```python
from build123d import *

# Parameters (mm, degrees)
SKETCH1_W                    = 44
SKETCH1_H                    = 90
BASE_FLANGE1_DEPTH           = 1.5
EDGE_FLANGE1_STRIP_W         = 7.4732
EDGE_FLANGE1_STRIP_H         = 1.5
EDGE_FLANGE1_STRIP_CUT_DEPTH = 90
EDGE_FLANGE1_DEPTH           = 90
EDGE_FLANGE2_STRIP_W         = 7.4732
EDGE_FLANGE2_STRIP_H         = 1.5
EDGE_FLANGE2_STRIP_CUT_DEPTH = 90
EDGE_FLANGE2_DEPTH           = 90
SKETCH12_R                   = 4.5
SKETCH12_R_2                 = 1.5
CUT_EXTRUDE4_DEPTH           = 68.906185285
SKETCH13_R                   = 4.5
SKETCH13_R_2                 = 1.5
CUT_EXTRUDE5_DEPTH           = 10
LPATTERN1_COUNT              = 2
LPATTERN1_PITCH              = 30
LPATTERN1_COL_COUNT          = 2
LPATTERN1_COL_PITCH          = 30
FILLET1_R                    = 2


# Sheet-metal steps are written as plain solids
with BuildPart() as part:
    # Sketch1 → Base-Flange1 (new body)
    with BuildSketch(Plane(origin=(0, 0, 0), x_dir=(1, 0, 0), z_dir=(0, 1, 0))):
        with Locations((-22, 0)):
            Rectangle(SKETCH1_W, SKETCH1_H)
    extrude(amount=BASE_FLANGE1_DEPTH)

    # Edge-Flange1 strip (across the edge) → Edge-Flange1 strip cut (cut)
    with BuildSketch(Plane(origin=(0, 1.5, 45), x_dir=(-1, 0, 0), z_dir=(0, 0, -1))):
        with Locations((-1.5, -0.75)):
            Rectangle(EDGE_FLANGE1_STRIP_W, EDGE_FLANGE1_STRIP_H)
    extrude(amount=EDGE_FLANGE1_STRIP_CUT_DEPTH, mode=Mode.SUBTRACT)

    # Edge-Flange1 section (across the edge) → Edge-Flange1 (add)
    with BuildSketch(Plane(origin=(0, 1.5, 45), x_dir=(-1, 0, 0), z_dir=(0, 0, -1))):
        with BuildLine():
            Line((0, 0.7366), (0, 24))
            Line((0, 24), (1.5, 24))
            Line((1.5, 24), (1.5, 0.7366))
            ThreePointArc((1.5, 0.7366), (1.715745145, 0.215745145), (2.2366, 0))
            Line((2.2366, 0), (2.2366, -1.5))
            ThreePointArc((2.2366, -1.5), (0.655084973, -0.844915027), (0, 0.7366))
        make_face()
    extrude(amount=EDGE_FLANGE1_DEPTH)

    # Edge-Flange2 strip (across the edge) → Edge-Flange2 strip cut (cut)
    with BuildSketch(Plane(origin=(-1.5, 25.5, 45), x_dir=(0, -1, 0), z_dir=(0, 0, -1))):
        with Locations((-1.5, -0.75)):
            Rectangle(EDGE_FLANGE2_STRIP_W, EDGE_FLANGE2_STRIP_H)
    extrude(amount=EDGE_FLANGE2_STRIP_CUT_DEPTH, mode=Mode.SUBTRACT)

    # Edge-Flange2 section (across the edge) → Edge-Flange2 (add)
    with BuildSketch(Plane(origin=(-1.5, 25.5, 45), x_dir=(0, -1, 0), z_dir=(0, 0, -1))):
        with BuildLine():
            Line((0, 0.7366), (0, 42.5))
            Line((0, 42.5), (1.5, 42.5))
            Line((1.5, 42.5), (1.5, 0.7366))
            ThreePointArc((1.5, 0.7366), (1.715745145, 0.215745145), (2.2366, 0))
            Line((2.2366, 0), (2.2366, -1.5))
            ThreePointArc((2.2366, -1.5), (0.655084973, -0.844915027), (0, 0.7366))
        make_face()
    extrude(amount=EDGE_FLANGE2_DEPTH)

    # Sketch12 → Cut-Extrude4 (cut, through all)
    with BuildSketch(Plane(origin=(0, 0, 0), x_dir=(1, 0, 0), z_dir=(0, 1, 0))):
        with Locations((-31, 35)):
            Circle(SKETCH12_R)
        with Locations((-31, 42)):
            Circle(SKETCH12_R_2)
        with Locations((-31, 28)):
            Circle(SKETCH12_R_2)
        with Locations((-24, 35)):
            Circle(SKETCH12_R_2)
        with Locations((-38, 35)):
            Circle(SKETCH12_R_2)
        with Locations((-31, 0)):
            Circle(SKETCH12_R)
        with Locations((-31, 7)):
            Circle(SKETCH12_R_2)
        with Locations((-31, -7)):
            Circle(SKETCH12_R_2)
        with Locations((-24, 0)):
            Circle(SKETCH12_R_2)
        with Locations((-38, 0)):
            Circle(SKETCH12_R_2)
        with Locations((-31, -35)):
            Circle(SKETCH12_R)
        with Locations((-31, -28)):
            Circle(SKETCH12_R_2)
        with Locations((-24, -35)):
            Circle(SKETCH12_R_2)
        with Locations((-38, -35)):
            Circle(SKETCH12_R_2)
        with Locations((-31, -42)):
            Circle(SKETCH12_R_2)
    extrude(amount=CUT_EXTRUDE4_DEPTH, mode=Mode.SUBTRACT)

    # Sketch13 → Cut-Extrude5 (cut)
    with BuildSketch(Plane.ZY.offset(1.5)):
        with Locations(Location((0, 12.75, 0), (0, 0, 270))):
            Circle(SKETCH13_R)
        with Locations(Location((0, 19.75, 0), (0, 0, 270))):
            Circle(SKETCH13_R_2)
        with Locations(Location((0, 5.75, 0), (0, 0, 270))):
            Circle(SKETCH13_R_2)
        with Locations(Location((7, 12.75, 0), (0, 0, 270))):
            Circle(SKETCH13_R_2)
        with Locations(Location((-7, 12.75, 0), (0, 0, 270))):
            Circle(SKETCH13_R_2)
    cut_extrude5 = extrude(amount=-CUT_EXTRUDE5_DEPTH, mode=Mode.SUBTRACT)

    # LPattern1: Cut-Extrude5 ×2
    with Locations(*[(0, 0, -i * LPATTERN1_PITCH) for i in range(1, LPATTERN1_COUNT)]):
        add(cut_extrude5, mode=Mode.SUBTRACT)

    # LPattern1 col: Cut-Extrude5 ×2
    with Locations(*[(0, 0, i * LPATTERN1_COL_PITCH) for i in range(1, LPATTERN1_COL_COUNT)]):
        add(cut_extrude5, mode=Mode.SUBTRACT)

    # Fillet1
    fillet1_edges = [part.edges().sort_by_distance(p)[0] for p in [
        (-44, 24.75, 45),
        (-44, 24.75, -45),
        (-44, 0.75, 45),
        (-44, 0.75, -45),
    ]]
    fillet(fillet1_edges, radius=FILLET1_R)


solid = part.part
```
Could you check a few things on this model? Use its own coordinates, in mm. Round coordinates to 2 decimals unless told otherwise and drop trailing zeros. Order: outer loops, then holes, each group sorted by start corner. A loop starts at its lowest first (then second) coordinate and runs counter-clockwise, first axis right, second up. Notation, with made-up numbers: (-4.75, 57) -> (23.25, 57) arc R12 ccw to (23.25, 67) -> close; hole circle Ø3 at (-26, -26.75). An arc over 180 degrees is marked (long way). One line per question, with ' | ' between items.
Q1. If we section it at B-B on x = -18.5: Write out the boundary of the cut face in (y, z).
Computed values:
outline: (0, -45) -> (1.5, -45) -> (1.5, 45) -> (0, 45) -> close; (24, -45) -> (25.5, -45) -> (25.5, 45) -> (24, 45) -> close
Q2. We'd pull the mould along Y, two halves only. Please class faces 1 (the face through (-0.64, 24.83, 0.63)), 2 (the face through (-0.76, 6.86, 31.01)), 3 (the face through (-28.92, 24.74, 38.99)): released by +Y, released by -Y, zero draft, split by the parting line, or undercut.
Computed values:
face 1: released by +Y | face 2: undercut | face 3: zero draft
Q3. If we section it at D-D on y = 10: Write out the boundary of the cut face in (x, z).
Computed values:
outline: (-1.5, -45) -> (0, -45) -> (0, -33.56) -> (-1.5, -33.56) -> close; (-1.5, -26.44) -> (0, -26.44) -> (0, -3.56) -> (-1.5, -3.56) -> close; (-1.5, 3.56) -> (0, 3.56) -> (0, 26.44) -> (-1.5, 26.44) -> close; (-1.5, 33.56) -> (0, 33.56) -> (0, 45) -> (-1.5, 45) -> close
Q4. If I drill on line 1 (Y direction, x = -37.5, z = 21); line 2 (X direction, y = 5.25, z = -21); line 3 (X direction, y = 23.75, z = -31.5), over which ranges is the centre line in solid material (lowest first)? Write a range as from..to.
Computed values:
line 1: 0..1.5, 24..25.5 | line 2: -1.5..0 | line 3: -1.68..-0.05
Q5. If we section it at A-A on z = 7: Write out the boundary of the cut face in (x, y).
Computed values:
outline: (-44, 0) -> (-32.5, 0) -> (-32.5, 1.5) -> (-44, 1.5) -> close; (-44, 24) -> (-32.5, 24) -> (-32.5, 25.5) -> (-44, 25.5) -> close; (-29.5, 0) -> (-2.24, 0) arc R2.24 ccw to (0, 2.24) -> (0, 11.25) -> (-1.5, 11.25) -> (-1.5, 2.24) arc R0.74 cw to (-2.24, 1.5) -> (-29.5, 1.5) -> close; (-29.5, 24) -> (-2.24, 24) arc R0.74 cw to (-1.5, 23.26) -> (-1.5, 14.25) -> (0, 14.25) -> (0, 23.26) arc R2.24 ccw to (-2.24, 25.5) -> (-29.5, 25.5) -> close
Q6. I'm going to push a flat-ended pin straight in: pin 1 (11.5 mm diameter, centred on y = 12.75, z = 0, fed in from -X). Where does the tip first touch, or does it pass through?
Computed values:
pin 1: x = -1.5
Q7. If we section it at C-C on x = -38: Give the number of separate pieces and of enclosed holes in the cut face, plus the area to 3 significant figures.
Computed values:
separate pieces: 8 | enclosed holes: 0 | area: 243 mm²
